Geometry: final body of the model. Coordinates: model frame, mm. A direction names the side the tool comes from. Round coordinates to 2 decimals unless told otherwise and drop trailing zeros. Order: outer loops, then holes, each group sorted by start corner. A loop starts at its lowest first (then second) coordinate and runs counter-clockwise, first axis right, second up. Notation, with made-up numbers: (-25, 14) -> (-17, 14) arc R15 ccw to (-17, 36) -> close; hole circle Ø3 at (61, -1). An arc over 180 degrees is marked (long way). Put each result on its own line as item: value.
```python
from build123d import *

# Parameters (mm, degrees)
FASE1_SIZE = 0.1


with BuildPart() as part:
    # Skizze2 → Rotation1 (revolve)
    with BuildSketch(Plane(origin=(0, 0, 0), x_dir=(0, 0, -1), z_dir=(1, 0, 0))):
        Polygon((-1.5, 2), (1.5, 2), (1.5, 2.5), (1, 2.5), (1, 3.4), (1.5, 3.4), (1.5, 4), (-1.5, 4), (-1.5, 3.4), (-1, 3.4), (-1, 2.5), (-1.5, 2.5), align=None)
    revolve(axis=Axis((0, 0, 11.845846522), (0, 0, -1)))

    # Fase1
    fase1_edges = [part.edges().sort_by_distance(p)[0] for p in [
        (0, -4, 1.5),
        (0, -4, -1.5),
        (0, -2, -1.5),
        (0, -2, 1.5),
    ]]
    chamfer(fase1_edges, length=FASE1_SIZE)


solid = part.part
```
1. Cut plane A-A on z = -1.3. Return loops of the section in (x, y), and give its area (3 significant figures).
Ans:
outline: circle Ø8 at (0, 0); circle Ø5 at (0, 0); hole circle Ø6.8 at (0, 0); hole circle Ø4 at (0, 0)
area: 21.0 mm²
2. Set-up query: faces 1 (the face through (3, 2, 1.5)), 2 (the face through (2, 2, -1)), 3 (the face through (-2.44, -0.54, 1.25)). Return all of +Z, -Z, +X, -X, +Y, -Y with unobstructed straight access to the full face (end or side cutting, diameter ignored); none if empty.
Ans:
face 1: +Z, +X, -X, +Y, -Y
face 2: -Z
face 3: +Z
3. Cut plane D-D on z = 0.9. Return loops of the section in (x, y), and give its area (3 significant figures).
Ans:
outline: circle Ø8 at (0, 0); hole circle Ø4 at (0, 0)
area: 37.7 mm²
4. Contact query for flat-ended pins moving along their axis: P1, Ø1, axis at y = -1, z = 1, coming from the -X side; P2, Ø4, axis at x = -0.5, y = -2.5, coming from the -Z side. Output: stop coordinate, or through.
Ans:
P1: x = -3.97
P2: z = -1.5
5. Draft query along Y for faces 4 (the face through (-3.905, -0.867, 0.02)), 5 (the face through (3, -2, -1.5)), 6 (the face through (-2.44, -0.54, -1.25)). Return one class per face: +Y half, -Y half, draft (parallel to the pull), parting line (faces both ways), or undercut.
Ans:
face 4: parting line
face 5: draft
face 6: undercut
6. Material intervals for probe 1 along X at (y, z) = (0, 1.35); probe 2 along Y at (x, z) = (-1.75, 1.1); probe 3 along Y at (x, z) = (0.5, -1.25), sorted ascending.
Ans:
probe 1: -4 to -3.4, -2.5 to -2, 2 to 2.5, 3.4 to 4
probe 2: -3.6 to -2.92, -1.79 to -0.97, 0.97 to 1.79, 2.92 to 3.6
probe 3: -3.97 to -3.36, -2.45 to -1.94, 1.94 to 2.45, 3.36 to 3.97
